Can you work these out from the model? Positions are in its coordinate system, mm. Face numbers are marked on the shaded views. A direction names the side the tool comes from. Coordinates: 2 decimals unless noted, no trailing zeros. Write item = value, one per line.
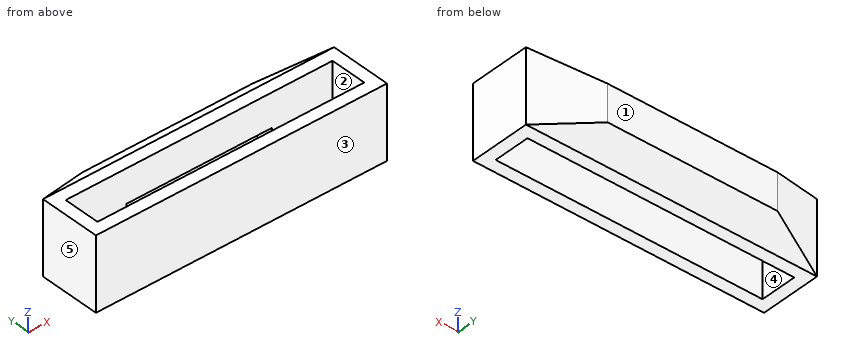
```python
from build123d import *

# Parameters (mm, degrees)
SKETCH1_W           = 24
SKETCH1_H           = 5
SKETCH1_W_2         = 22
SKETCH1_H_2         = 3
BOSS_EXTRUDE1_DEPTH = 6
SKETCH2_W           = 14
SKETCH2_H           = 3
SKETCH5_R           = 1.25
CUT_EXTRUDE1_DEPTH  = 6


with BuildPart() as part:
    # Sketch1 → Boss-Extrude1 (new body)
    with BuildSketch(Plane.XY):
        with Locations((0, 2.5)):
            Rectangle(SKETCH1_W, SKETCH1_H)
        with Locations((0, 2.5)):
            Rectangle(SKETCH1_W_2, SKETCH1_H_2, mode=Mode.SUBTRACT)
    extrude(amount=BOSS_EXTRUDE1_DEPTH)

    # Sketch2 → section 1 of loft1
    with BuildSketch(Plane(origin=(0, 7, 0), x_dir=(1, 0, 0), z_dir=(0, 1, 0)), mode=Mode.PRIVATE) as loft1_s1:
        with Locations((0, -3)):
            Rectangle(SKETCH2_W, SKETCH2_H)
    # loft from a face of the part (loft1)
    loft([part.faces().sort_by_distance((0, 5, 3))[0], loft1_s1.sketch])

    # Sketch5 → Cut-Extrude1 (cut, symmetric)
    with BuildSketch(Plane(origin=(0, 0, 0), x_dir=(0, 0, -1), z_dir=(1, 0, 0))):
        with Locations((-3, 5.224744871)):
            Circle(SKETCH5_R)
    extrude(amount=CUT_EXTRUDE1_DEPTH, both=True, mode=Mode.SUBTRACT)


solid = part.part
```
Item 1: If we mould it in two halves opening along Y, with no side actions, what happens to the marked faces 1, 2 and 3? For each: pulls with the +Y half, pulls with the -Y half, needs draft (parallel to the pull), parting line crosses it, or undercut.
A:
face_1 = pulls with the +Y half
face_2 = undercut
face_3 = pulls with the -Y half
Item 2: I'm going to push a flat-ended pin straight in: P1, Ø2, axis at y = 5.22, z = 3, coming from the +X side. Where does the tip first touch, or does it pass through?
A:
P1 = 12
Item 3: If I drill on probe 1 along X at (y, z) = (1.5, 4.75); probe 2 along Y at (x, z) = (3, 3); probe 3 along X at (y, z) = (4.75, 2.5), over which ranges is the centre line in solid material (lowest first)?
A:
probe_1 = -12 to -11, 11 to 12
probe_2 = 0 to 1, 6.47 to 7
probe_3 = -12 to -6, 6 to 12
Item 4: For the marked faces 4 and 5, which set-ups out of +Z, -Z, +X, -X, +Y, -Y let a thin tool reach every point of the face, with its end or its side?
A:
face_4 = +Z, -Z
face_5 = +Z, -Z, -X, +Y, -Y
Item 5: I want a section at A-A, the plane z = 2. Give the number of separate pieces and of enclosed holes in the cut face, plus the area to 3 significant figures.
A:
separate_pieces = 1
enclosed_holes = 2
area = 74.0 mm2
